Autodesk Inventor part; units mm, degrees
ref_plane "YZ Plane" through (0, 0, 0) normal (1, 0, 0) x (0, 1, 0)
ref_plane "XZ Plane" through (0, 0, 0) normal (0, 1, 0) x (-1, 0, 0)
ref_plane "XY Plane" through (0, 0, 0) normal (0, 0, 1) x (1, 0, 0)
sketch "Sketch1" plane through (0, 0, 0) normal (0, 1, 0) x (-1, 0, 0)
  point P0 (0, 0)
sketch "Sketch2" plane through (0, 0, 0) normal (0, 1, 0) x (-1, 0, 0)
  line L0 (0, 0) -> (0, -7.5)
  line L1 (0, -7.5) -> (75, -7.5)
  line L2 (75, -7.5) -> (75, 7.5)
  line L3 (75, 7.5) -> (0, 7.5)
  line L4 (0, 7.5) -> (0, 0)
  arc A0 (0, 7.5) -> (0, -7.5) centre (0, 0) ccw
  dimension "d0" = 7.5
  dimension "d1" = 75
  dimension "d2" = 15
extrude "Extrusion1" add sketch "Sketch2" along normal blind 10
sketch "Sketch3" plane through (0, 10, 0) normal (0, 1, 0) x (1, 0, 0)
  point P0 (0, 0)
  point P1 (0, 0)
hole "Hole1" at (0, 10, 0) direction (0, -1, 0) diameter 10 end through all
sketch "Sketch4" plane through (-75, 0, -7.5) normal (-1, 0, 0) x (0, 0, 1)
  circle A0 centre (7.5, 5) radius 2.5
  point P0 (7.5, 0)
  dimension "d14" = 5
extrude "Extrusion2" add sketch "Sketch4" along normal blind 20
properties part number "Arm"
CAD build for the part. Positions are in the model's coordinates, mm. A direction names the side the tool comes from. Round coordinates to 2 decimals unless told otherwise and drop trailing zeros. Loops run counter-clockwise (first coordinate to the right, second up) from the corner with the lowest first, then second, coordinate; pieces in that order, holes last. Notation, with made-up numbers: M -0.5,14.5 L 43.5,14.5 A24 cw 43.5,31.5 Z; hole C -11,-3 d3. An arc over 180 degrees is marked long. Return JSON: item names as keys, results as strings. Group by question number.
(1) Mould opens along Z. For faces 1 (the flat face through (-37, 5, -7.5)), 2 (the cylindrical face through (4.88, 4.93, -1.08)), 3 (the flat face through (-38, 5, 7.5)) say: +Z half, -Z half, draft (parallel to the pull), parting line (faces both ways), or undercut.
(2) Saw through at A-A, the plane z = 0. List the corners of the cut face in (x, y).
(3) Saw through at C-C, the plane x = -82. List the corners of the cut face in (y, z).
(4) Saw through at B-B, the plane y = 6.25. List the corners of the cut face in (x, z).
(5) Saw through at D-D, the plane z = 4. List the corners of the cut face in (x, y), and give its area (3 significant figures).
(6) Wall check: probe 1 along X at (y, z) = (6.75, 0); probe 2 along Z at (x, y) = (0, 3); probe 3 along Y at (x, z) = (-86, 0.25). Give the ranges that are in metal, low to high. Write a range as [from, to].
(7) Tool access for faces 4 (the flat face through (-33, 10, 0)), 5 (the cylindrical face through (-84.86, 2.52, -0.33)): list every direction of +Z, -Z, +X, -X, +Y, -Y with a clear straight run to the whole face (end or side of a thin tool).
Answer list:
{
 "1": {"face 1": "-Z half", "face 2": "undercut", "face 3": "+Z half"},
 "2": {"outline": "M -95,2.5 L -75,2.5 L -75,0 L -5,0 L -5,10 L -75,10 L -75,7.5 L -95,7.5 Z; M 5,0 L 7.5,0 L 7.5,10 L 5,10 Z"},
 "3": {"outline": "C 5,0 d5"},
 "4": {"outline": "M -95,-2.17 L -75,-2.17 L -75,-7.5 L 0,-7.5 A7.5 ccw 0,7.5 L -75,7.5 L -75,2.17 L -95,2.17 Z; hole C 0,0 d10"},
 "5": {"outline": "M -75,0 L -3,0 L -3,10 L -75,10 Z; M 3,0 L 6.34,0 L 6.34,10 L 3,10 Z", "area": "753 mm2"},
 "6": {"probe 1": "[-95, -5], [5, 7.5]", "probe 2": "[-7.5, -5], [5, 7.5]", "probe 3": "[2.51, 7.49]"},
 "7": {"face 4": "+Z, -Z, +X, -X, +Y", "face 5": "-X"}
}
